Could you check a few things on this model? Use its own coordinates, in mm. A direction names the side the tool comes from. Coordinates: 2 decimals unless noted, no trailing zeros. Order: outer loops, then holes, each group sorted by start corner. A loop starts at its lowest first (then second) coordinate and runs counter-clockwise, first axis right, second up. Notation, with made-up numbers: (18.25, 89.5) -> (62.25, 89.5) arc R12 cw to (62.25, 100.5) -> close; hole circle Ø6 at (55.5, -27). An arc over 180 degrees is marked (long way). Put each result on its own line as item: value. Start each with the question number.
Q1. Will these pins go through, and if not, where does the flat tip stop? pin 1 (12 mm diameter, centred on y = 98.5, z = -8, fed in from -X); pin 2 (8 mm diameter, centred on y = 64, z = -29.5, fed in from +X); pin 3 (25 mm diameter, centred on x = -247.5, y = 147.5, fed in from +Z).
Q2. Please list where these lines run through material, in increasing order: line 1 along X through (y, z) = (103, -30.5); line 2 along Z through (x, y) = (-263, 51.5); line 3 along Z through (x, y) = (-244, 164.5).
Q3. If we section it at C-C (z = -26.5): Please give me the cut outline in (x, y).
Q4. For faces 4 (the face through (-369, 183, -40)), 5 (the face through (-289, 68, -10)), 6 (the face through (-243, 180, -40)), 7 (the face through (-235.21, 41.16, -42.46)), 8 (the face through (-307, 33.848, -42)), which set-ups out of +Z, -Z, +X, -X, +Y, -Y let a thin tool reach every point of the face, with its end or its side?
Q5. If we section it at B-B (z = -8): Please give me the cut outline in (x, y), and give its area (3 significant figures).
Q6. If we section it at A-A (z = -42): Please give me the cut outline in (x, y).
Q7. We'd pull the mould along Y, two halves only. Please class faces 1 (the face through (-306, 117, 0)), 2 (the face through (-246.7, 92.5, -15.1)), 3 (the face through (-225.73, 37.05, -42.46)): +Y half, -Y half, draft (parallel to the pull), parting line (faces both ways), or undercut.
from build123d import *

# Parameters (mm, degrees)
SKETCH4_R           = 45
BOSS_EXTRUDE1_DEPTH = 10
BOSS_EXTRUDE1_DRAFT = 29
SKETCH7_R           = 59.508676161
BOSS_EXTRUDE2_DEPTH = 30
BOSS_EXTRUDE2_DRAFT = 38
FILLET1_R           = 10
SKETCH9_W           = 165.894489912
SKETCH9_H           = 165.894489912
BOSS_EXTRUDE3_DEPTH = 5


with BuildPart() as part:
    # Sketch4 → Boss-Extrude1 (with draft: the straight prism first)
    with BuildSketch(Plane.XY):
        with Locations((-305.359774759, 116.794851209)):
            Circle(SKETCH4_R)
    extrude(amount=-BOSS_EXTRUDE1_DEPTH)
    # Boss-Extrude1: the draft: its side faces are tilted about the plane it starts from
    boss_extrude1_sides = [part.faces().sort_by_distance(p)[0] for p in [
        (-350.359774759, 116.794851209, -5),
    ]]
    draft(boss_extrude1_sides, Plane.XY, BOSS_EXTRUDE1_DRAFT)


with BuildPart() as boss_extrude2_tool:
    # Sketch7 → Boss-Extrude2 (with draft: the straight prism first)
    with BuildSketch(Plane.XY.offset(-10)):
        with Locations((-305.359774759, 116.794851209)):
            Circle(SKETCH7_R)
    extrude(amount=-BOSS_EXTRUDE2_DEPTH)
    # Boss-Extrude2: the draft: its side faces are tilted about the plane it starts from
    boss_extrude2_sides = [boss_extrude2_tool.faces().sort_by_distance(p)[0] for p in [
        (-364.868450919, 116.794851209, -25),
    ]]
    draft(boss_extrude2_sides, Plane.XY.offset(-10), BOSS_EXTRUDE2_DRAFT)


with BuildPart() as part_1:
    add(part.part)

    # Boss-Extrude2: add boss_extrude2_tool
    add(boss_extrude2_tool.part)

    # Fillet1
    fillet1_edges = [part_1.edges().sort_by_distance(p)[0] for p in [
        (-364.868450919, 116.794851209, -10),
    ]]
    fillet(fillet1_edges, radius=FILLET1_R)

    # Sketch9 → Boss-Extrude3 (add)
    with BuildSketch(Plane.XY.offset(-40)):
        with Locations((-305.359774759, 116.794851209)):
            Rectangle(SKETCH9_W, SKETCH9_H)
        with BuildLine():
            Line((-225.670814758, 191.00038112), (-233.670814758, 183.00038112))
            ThreePointArc((-233.670814758, 183.00038112), (-239.154244847, 183.00038112), (-239.154244847, 188.48381121))
            Line((-239.154244847, 188.48381121), (-231.154244847, 196.48381121))
            ThreePointArc((-231.154244847, 196.48381121), (-225.670814758, 196.48381121), (-225.670814758, 191.00038112))
        make_face(mode=Mode.SUBTRACT)
        with BuildLine():
            Line((-385.048734759, 191.00038112), (-377.048734759, 183.00038112))
            ThreePointArc((-377.048734759, 183.00038112), (-371.56530467, 183.00038112), (-371.56530467, 188.48381121))
            Line((-371.56530467, 188.48381121), (-379.56530467, 196.48381121))
            ThreePointArc((-379.56530467, 196.48381121), (-385.048734759, 196.48381121), (-385.048734759, 191.00038112))
        make_face(mode=Mode.SUBTRACT)
        with BuildLine():
            Line((-385.048734759, 42.589321298), (-377.048734759, 50.589321298))
            ThreePointArc((-377.048734759, 50.589321298), (-371.56530467, 50.589321298), (-371.56530467, 45.105891208))
            Line((-371.56530467, 45.105891208), (-379.56530467, 37.105891208))
            ThreePointArc((-379.56530467, 37.105891208), (-385.048734759, 37.105891208), (-385.048734759, 42.589321298))
        make_face(mode=Mode.SUBTRACT)
        with BuildLine():
            Line((-225.670814758, 42.589321298), (-233.670814758, 50.589321298))
            ThreePointArc((-233.670814758, 50.589321298), (-239.154244847, 50.589321298), (-239.154244847, 45.105891208))
            Line((-239.154244847, 45.105891208), (-231.154244847, 37.105891208))
            ThreePointArc((-231.154244847, 37.105891208), (-225.670814758, 37.105891208), (-225.670814758, 42.589321298))
        make_face(mode=Mode.SUBTRACT)
    extrude(amount=-BOSS_EXTRUDE3_DEPTH)


solid = part_1.part
The answers:
1. pin 1: x = -365.56
1. pin 2: x = -246.81
1. pin 3: z = -10
2. line 1: -379.61 to -231.11
2. line 2: -45 to -33.45
2. line 3: -45 to -33.31
3. outline: circle Ø144.8 at (-305.36, 116.79)
4. face 4: +Z, -X, +Y
4. face 5: +Z
4. face 6: +Z, +X, +Y
4. face 7: +Z, -Z
4. face 8: +Z, -Z, +X, -X, -Y
5. outline: circle Ø98.87 at (-305.36, 116.79)
5. area: 7,680 mm^2
6. outline: (-388.31, 33.85) -> (-222.41, 33.85) -> (-222.41, 199.74) -> (-388.31, 199.74) -> close; hole (-385.05, 42.59) arc R3.88 ccw to (-379.57, 37.11) -> (-371.57, 45.11) arc R3.88 ccw to (-377.05, 50.59) -> close; hole (-385.05, 191) -> (-377.05, 183) arc R3.88 ccw to (-371.57, 188.48) -> (-379.57, 196.48) arc R3.88 ccw to start; hole (-239.15, 45.11) -> (-231.15, 37.11) arc R3.88 ccw to (-225.67, 42.59) -> (-233.67, 50.59) arc R3.88 ccw to start; hole (-239.15, 188.48) arc R3.88 ccw to (-233.67, 183) -> (-225.67, 191) arc R3.88 ccw to (-231.15, 196.48) -> close
7. face 1: draft
7. face 2: parting line
7. face 3: undercut
